from build123d import *

# Parameters (mm, degrees)
BOSS_EXTRUDE1_DEPTH = 1.524
SKETCH2_W           = 12.7
SKETCH2_H           = 1.537730424
SKETCH2_H_2         = 1.537730425
CUT_EXTRUDE1_DEPTH  = 1.524


with BuildPart() as part:
    # Sketch1 → Boss-Extrude1 (new body)
    with BuildSketch(Plane.XY):
        Polygon((-102.477755775, -1.524), (-110.726395883, -58.314338926), (-126.787898899, -58.314338926), (-126.787898899, -59.838338926), (-133.137898899, -59.838338926), (-133.137898899, -58.314338926), (-149.199401915, -58.314338926), (-149.6392871, -1.524), (-129.233521437, -1.524), (-129.233521437, 1.524), (-130.821021437, 1.524), (-130.821021437, 3.048), (-121.296021437, 3.048), (-121.296021437, 1.524), (-122.883521437, 1.524), (-122.883521437, -1.524), align=None)
    extrude(amount=BOSS_EXTRUDE1_DEPTH)

    # Sketch2 → Cut-Extrude1 (cut)
    with BuildSketch(Plane.XY.offset(1.524)):
        with Locations((-127.078752717, -17.602011312)):
            Rectangle(SKETCH2_W, SKETCH2_H)
        with Locations((-127.078752717, -40.703047377)):
            Rectangle(SKETCH2_W, SKETCH2_H_2)
    extrude(amount=-CUT_EXTRUDE1_DEPTH, mode=Mode.SUBTRACT)


solid = part.part
Build history of the part. All positions in model axes, mm. A direction names the side the tool comes from. Give positions to 0.01 mm unless a question says otherwise; leave off trailing zeros. Write each loop counter-clockwise with the first axis right and the second up, starting at its lowest first coordinate (ties: lowest second). Pieces come first, ordered by that corner, then holes. Notation, with made-up numbers: (77, 41.25) - (123, 41.25) arc R9 cw to (123, 56.25) - close; hole circle Ø1 at (-8.5, 48.5). An arc over 180 degrees is marked (long way). Use one line per item in the form item = value. Start each with the question number.
1. 3-axis set-ups, long thin cutter, end or side, ignore diameter. For faces 5 (the face through (-127, -39.934, 1)), 6 (the face through (-122.884, 0, 1)), 7 (the face through (-129.234, 0, 1)), 8 (the face through (-126.788, -59, 1)): which of +Z, -Z, +X, -X, +Y, -Y reach the whole face in a straight line?
2. Drop flat-ended pins along their axis: pin 1 Ø0.8 at (y, z) = (0.5, 0.5) entering from +X; pin 2 Ø0.5 at (x, z) = (-141.5, 1) entering from -Y; pin 3 Ø0.5 at (y, z) = (-17.5, 1) entering from -X. Give the stop position or say it passes through.
3. Band-saw the part on C-C on y = -12. Write the cut outline in (x, z).
4. Band-saw the part on A-A on z = 0.7. Write the cut outline in (x, y).
5. Two-plate mould, pull along Y, no slides. Class faces 1 (the face through (-130.821, 2, 1)), 2 (the face through (-141, -58.314, 1)), 3 (the face through (-133.429, -18, 1)), 4 (the face through (-130, 1.524, 1)): released by +Y, released by -Y, zero draft, split by the parting line, or undercut.
6. Band-saw the part on B-B on x = -141. Write the cut outline in (y, z), plus the area to 3 significant figures.
7. Probe line 1 (Y direction, x = -124, z = 0.3); line 2 (Y direction, x = -128.5, z = 0.2); line 3 (Y direction, x = -136.5, z = 0.1). List the from-to ranges inside material, lowest first. Write a range as [from, to].
Conclusion:
q1.face_5 = +Z, -Z
q1.face_6 = +Z, -Z, +X
q1.face_7 = +Z, -Z, -X
q1.face_8 = +Z, -Z, +X, -Y
q2.pin_1 = -122.88
q2.pin_2 = -58.31
q2.pin_3 = -149.52
q3.outline = (-149.56, 0) - (-104, 0) - (-104, 1.52) - (-149.56, 1.52) - close
q4.outline = (-149.64, -1.52) - (-149.2, -58.31) - (-133.14, -58.31) - (-133.14, -59.84) - (-126.79, -59.84) - (-126.79, -58.31) - (-110.73, -58.31) - (-102.48, -1.52) - (-122.88, -1.52) - (-122.88, 1.52) - (-121.3, 1.52) - (-121.3, 3.05) - (-130.82, 3.05) - (-130.82, 1.52) - (-129.23, 1.52) - (-129.23, -1.52) - close; hole (-133.43, -41.47) - (-120.73, -41.47) - (-120.73, -39.93) - (-133.43, -39.93) - close; hole (-133.43, -18.37) - (-120.73, -18.37) - (-120.73, -16.83) - (-133.43, -16.83) - close
q5.face_1 = zero draft
q5.face_2 = released by -Y
q5.face_3 = undercut
q5.face_4 = undercut
q6.outline = (-58.31, 0) - (-1.52, 0) - (-1.52, 1.52) - (-58.31, 1.52) - close
q6.area = 86.5 mm²
q7.line_1 = [-58.31, -41.47], [-39.93, -18.37], [-16.83, 3.05]
q7.line_2 = [-59.84, -41.47], [-39.93, -18.37], [-16.83, 3.05]
q7.line_3 = [-58.31, -1.52]
